Autodesk Inventor part; units mm, degrees
ref_plane "YZ Plane" through (0, 0, 0) normal (1, 0, 0) x (0, 1, 0)
ref_plane "XZ Plane" through (0, 0, 0) normal (0, 1, 0) x (-1, 0, 0)
ref_plane "XY Plane" through (0, 0, 0) normal (0, 0, 1) x (1, 0, 0)
sketch "スケッチ1" plane through (0, 0, 0) normal (0, 0, 1) x (1, 0, 0)
  circle A0 centre (0, 0) radius 2
  dimension "d0" = 4
extrude "押し出し1" add sketch "スケッチ1" along normal blind 8
sketch "スケッチ2" plane through (0, 0, 0) normal (0, 0, -1) x (-1, 0, 0)
  circle A0 centre (0, 0) radius 4
  dimension "d3" = 8
extrude "押し出し2" add sketch "スケッチ2" along normal blind 1.5
thread "ねじ1"
chamfer "面取り1" distance 0.5 angle 30 1 edges at (4, 0, -1.5) measured on face at (-0.7574, 1.0973, -1.5)
properties part number "ネジローヘッドm4,08" material "鋼、高強度、低合金"
Can you work these out from the model? Positions are in its coordinate system, mm. A direction names the side the tool comes from. Round coordinates to 2 decimals unless told otherwise and drop trailing zeros. Write each loop counter-clockwise with the first axis right and the second up, starting at its lowest first coordinate (ties: lowest second). Pieces come first, ordered by that corner, then holes. Notation, with made-up numbers: M 31,50 L 46,50 A24 ccw 46,78 Z; hole C -26,20 d4. An arc over 180 degrees is marked long. Use a Markdown table: item, result.
Item 1: I want a section at C-C (z = 7). List the corners of the cut face in (x, y) for me, and give its area (3 significant figures).
Found:
| item | result |
|---|---|
| outline | C 0,0 d4 |
| area | 12.6 mm2 |
Item 2: If I drill on line 1 along Y through (x, z) = (0, 3.75); line 2 along Z through (x, y) = (-3, 1.75); line 3 along Z through (x, y) = (-1.75, -3.25), over which ranges is the centre line in solid material (lowest first)? Write a range as [from, to].
Found:
| item | result |
|---|---|
| line 1 | y = [-2, 2] |
| line 2 | z = [-1.5, 0] |
| line 3 | z = [-1.39, 0] |
Item 3: For pin 1 Ø4 at (x, z) = (-1.5, 7) entering from +Y; pin 2 Ø2 at (y, z) = (0, 5) entering from +X; pin 3 Ø3 at (y, z) = (-2.5, 3.5) entering from +X, each with a flat end and sliding along its axis, tell me the tip position at first contact or that it passes through.
Found:
| item | result |
|---|---|
| pin 1 | stops at y = 2 |
| pin 2 | stops at x = 2 |
| pin 3 | stops at x = 1.73 |
Item 4: Which directions (+Z, -Z, +X, -X, +Y, -Y) give clear straight access to the entire face, cutting with the end or side of a thin tool? Please do faces 1 (the face through (0, 2, 4)), 2 (the face through (0, 0, 8)).
Found:
| item | result |
|---|---|
| face 1 | +Z |
| face 2 | +Z, +X, -X, +Y, -Y |
Item 5: I want a section at A-A (y = 0). List the corners of the cut face in (x, z) for me, and give its area (3 significant figures).
Found:
| item | result |
|---|---|
| outline | M -4,-1.21 L -3.5,-1.5 L 3.5,-1.5 L 4,-1.21 L 4,0 L 2,0 L 2,8 L -2,8 L -2,0 L -4,0 Z |
| area | 43.9 mm2 |
